```python
from build123d import *

# Parameters (mm, degrees)
F0_W         = 55
F0_H         = 46
F5_DEPTH     = 70
F1_W         = 7.25
F1_H         = 70
F6_DEPTH     = 23
F7_D         = 6
F7_DEPTH     = 15
F7_TIP       = 1.8025818571
F9_DEPTH     = 4
F10_W        = 36
F10_H        = 36
F11_DEPTH    = 4
F12_D        = 6
F12_DEPTH    = 38
F12_TIP      = 1.8025818571
F14_DEPTH    = 4
F15_T1_DEPTH = 95
F16_DEPTH    = 33
F17_DEPTH    = 10


# Not quite as in the source:
# - a fillet or chamfer that OpenCascade refuses, or shapes differently, is made with other operations: its cross-section is extruded or revolved along the edge and cut away or added


with BuildPart() as f5:
    # F0 (on Front) → F5 (new body)
    with BuildSketch(Plane.XZ):
        Rectangle(F0_W, F0_H)
    extrude(amount=-F5_DEPTH)

    # F1 (on Top) → F6 (intersect, symmetric)
    with BuildSketch(Plane.XY):
        with BuildLine():
            Line((-20.25, 0), (-13, 0))
            ThreePointArc((-13, 0), (0, 13), (13, 0))
            Line((13, 0), (20.25, 0))
            Line((20.25, 0), (20.25, 70))
            Line((20.25, 70), (-20.25, 70))
            Line((-20.25, 70), (-20.25, 0))
        make_face()
        with Locations((-23.875, 35)):
            Rectangle(F1_W, F1_H)
        with Locations((23.875, 35)):
            Rectangle(F1_W, F1_H)
    extrude(amount=F6_DEPTH, both=True, mode=Mode.INTERSECT)

    # F7
    with Locations(Plane.XZ):
        with Locations((-20.25, 0), (20.25, 0)):
            Hole(F7_D / 2, depth=F7_DEPTH)
            with Locations((0, 0, -(F7_DEPTH + F7_TIP / 2))):  # 118° drill point
                Cone(0, F7_D / 2, F7_TIP, mode=Mode.SUBTRACT)

    # F8 (on offset) → F9 (cut)
    with BuildSketch(Plane.XZ.offset(-9)):
        Polygon((-24.5, 2.4537386441), (-24.5, 2.25), (-24.5, -2.4537386441), (-20.25, -4.9074772881), (-16, -2.4537386441), (-16, 2), (-16, 2.4537386441), (-20.25, 4.9074772881), align=None)
        Polygon((-24.5, 23), (-24.5, 2.4537386441), (-20.25, 4.9074772881), (-16, 2.4537386441), (-16, 23), align=None)
        Polygon((24.5, 2.4537386441), (24.5, 23), (16, 23), (16, 2.4537386441), (16, 2), (16, -2.4537386441), (20.25, -4.9074772881), (24.5, -2.4537386441), (24.5, 2.25), align=None)
    extrude(amount=-F9_DEPTH, mode=Mode.SUBTRACT)

    # F10 (on offset) → F11 (cut)
    with BuildSketch(Plane.XZ.offset(-66)):
        Rectangle(F10_W, F10_H)
    extrude(amount=-F11_DEPTH, mode=Mode.SUBTRACT)

    # F12
    with Locations(Plane(origin=(0, 66, 0), x_dir=(1, 0, 0), z_dir=(0, 1, 0))):
        with Locations((0, 0)):
            Hole(F12_D / 2, depth=F12_DEPTH)
            with Locations((0, 0, -(F12_DEPTH + F12_TIP / 2))):  # 118° drill point
                Cone(0, F12_D / 2, F12_TIP, mode=Mode.SUBTRACT)

    # F13 (on offset) → F14 (cut)
    with BuildSketch(Plane.XZ.offset(-29)):
        Polygon((-4.25, 2.4537386441), (-4.25, 2.25), (-4.25, -2.4537386441), (0, -4.9074772881), (4.25, -2.4537386441), (4.25, 2.0686155439), (4.25, 2.4537386441), (0, 4.9074772881), align=None)
        Polygon((-4.25, 23), (-4.25, 2.4537386441), (0, 4.9074772881), (4.25, 2.4537386441), (4.25, 23), align=None)
        with BuildLine():
            ThreePointArc((23.5, 14), (22.0355339059, 17.5355339059), (18.5, 19))
            Line((18.5, 19), (13.25, 19))
            ThreePointArc((13.25, 19), (9.7144660941, 17.5355339059), (8.25, 14))
            Line((8.25, 14), (8.25, -14))
            ThreePointArc((8.25, -14), (9.7144660941, -17.5355339059), (13.25, -19))
            Line((13.25, -19), (18.5, -19))
            ThreePointArc((18.5, -19), (22.0355339059, -17.5355339059), (23.5, -14))
            Line((23.5, -14), (23.5, 14))
        make_face()
        with BuildLine():
            Line((-13.25, 19), (-18.5, 19))
            ThreePointArc((-18.5, 19), (-22.0355339059, 17.5355339059), (-23.5, 14))
            Line((-23.5, 14), (-23.5, -14))
            ThreePointArc((-23.5, -14), (-22.0355339059, -17.5355339059), (-18.5, -19))
            Line((-18.5, -19), (-13.25, -19))
            ThreePointArc((-13.25, -19), (-9.7144660941, -17.5355339059), (-8.25, -14))
            Line((-8.25, -14), (-8.25, 14))
            ThreePointArc((-8.25, 14), (-9.7144660941, 17.5355339059), (-13.25, 19))
        make_face()
    extrude(amount=-F14_DEPTH, mode=Mode.SUBTRACT)

    # F15: fillet of radius 5 on 4 edges, made by hand

    # F15_s2 → F15_t1 (cut)
    with BuildSketch(Plane.XZ.offset(-82.5)):
        with BuildLine():
            ThreePointArc((-22.5, 23), (-26.0355339059, 21.5355339059), (-27.5, 18))
            Line((-27.5, 18), (-27.5, 23))
            Line((-27.5, 23), (-22.5, 23))
        make_face()
        with BuildLine():
            ThreePointArc((22.5, 23), (26.0355339059, 21.5355339059), (27.5, 18))
            Line((27.5, 18), (27.5, 23))
            Line((27.5, 23), (22.5, 23))
        make_face()
        with BuildLine():
            ThreePointArc((-22.5, -23), (-26.0355339059, -21.5355339059), (-27.5, -18))
            Line((-27.5, -18), (-27.5, -23))
            Line((-27.5, -23), (-22.5, -23))
        make_face()
        with BuildLine():
            ThreePointArc((22.5, -23), (26.0355339059, -21.5355339059), (27.5, -18))
            Line((27.5, -18), (27.5, -23))
            Line((27.5, -23), (22.5, -23))
        make_face()
    extrude(amount=F15_T1_DEPTH, mode=Mode.SUBTRACT)

    # F13 (on offset) → F16 (cut)
    with BuildSketch(Plane.XZ.offset(-29)):
        with BuildLine():
            ThreePointArc((23.5, 14), (22.0355339059, 17.5355339059), (18.5, 19))
            Line((18.5, 19), (13.25, 19))
            ThreePointArc((13.25, 19), (9.7144660941, 17.5355339059), (8.25, 14))
            Line((8.25, 14), (8.25, -14))
            ThreePointArc((8.25, -14), (9.7144660941, -17.5355339059), (13.25, -19))
            Line((13.25, -19), (18.5, -19))
            ThreePointArc((18.5, -19), (22.0355339059, -17.5355339059), (23.5, -14))
            Line((23.5, -14), (23.5, 14))
        make_face()
        with BuildLine():
            Line((-13.25, 19), (-18.5, 19))
            ThreePointArc((-18.5, 19), (-22.0355339059, 17.5355339059), (-23.5, 14))
            Line((-23.5, 14), (-23.5, -14))
            ThreePointArc((-23.5, -14), (-22.0355339059, -17.5355339059), (-18.5, -19))
            Line((-18.5, -19), (-13.25, -19))
            ThreePointArc((-13.25, -19), (-9.7144660941, -17.5355339059), (-8.25, -14))
            Line((-8.25, -14), (-8.25, 14))
            ThreePointArc((-8.25, 14), (-9.7144660941, 17.5355339059), (-13.25, 19))
        make_face()
    extrude(amount=-F16_DEPTH, mode=Mode.SUBTRACT)

    # F13 (on offset) → F17 (cut)
    with BuildSketch(Plane.XZ.offset(-29)):
        with BuildLine():
            ThreePointArc((23.5, 14), (22.0355339059, 17.5355339059), (18.5, 19))
            Line((18.5, 19), (13.25, 19))
            ThreePointArc((13.25, 19), (9.7144660941, 17.5355339059), (8.25, 14))
            Line((8.25, 14), (8.25, -14))
            ThreePointArc((8.25, -14), (9.7144660941, -17.5355339059), (13.25, -19))
            Line((13.25, -19), (18.5, -19))
            ThreePointArc((18.5, -19), (22.0355339059, -17.5355339059), (23.5, -14))
            Line((23.5, -14), (23.5, 14))
        make_face()
        with BuildLine():
            Line((-13.25, 19), (-18.5, 19))
            ThreePointArc((-18.5, 19), (-22.0355339059, 17.5355339059), (-23.5, 14))
            Line((-23.5, 14), (-23.5, -14))
            ThreePointArc((-23.5, -14), (-22.0355339059, -17.5355339059), (-18.5, -19))
            Line((-18.5, -19), (-13.25, -19))
            ThreePointArc((-13.25, -19), (-9.7144660941, -17.5355339059), (-8.25, -14))
            Line((-8.25, -14), (-8.25, 14))
            ThreePointArc((-8.25, 14), (-9.7144660941, 17.5355339059), (-13.25, 19))
        make_face()
    extrude(amount=F17_DEPTH, mode=Mode.SUBTRACT)


solid = f5.part
```
Geometry check sheet. Reference: the model listing, model coordinates, mm. A direction names the side the tool comes from. Give positions to 0.01 mm unless a question says otherwise; leave off trailing zeros. Order: outer loops, then holes, each group sorted by start corner. A loop starts at its lowest first (then second) coordinate and runs counter-clockwise, first axis right, second up. Notation, with made-up numbers: (-10, 45) - (-5, 45) arc R5 cw to (-5, 54) - close; hole circle Ø5 at (-32, 10.5). An arc over 180 degrees is marked (long way). Write item = value, one per line. Start each with the question number.
1) Section check C-C (x = -6.5). Enter the section's corners in (y, z), then the cut area to 3 significant figures.
2) Section check A-A (z = -11.5). Enter the section's corners in (x, y).
3) Gauge pin test, flat ends, axial feed: pin 1 Ø4 at (x, z) = (1.5, 7) entering from -Y; pin 2 Ø8 at (x, z) = (-10.5, -7) entering from +Y; pin 3 Ø4.5 at (x, z) = (17.5, -4.5) entering from +Y; pin 4 Ø5 at (x, z) = (0, 0) entering from -Y. Record the tip position at first contact, or that the pin passes through.
4) Access from +Z, -Z, +X, -X, +Y, -Y to the whole of each face (thin tool, end or side, straight path). Record for faces 1 (the flat face through (-18, 68, 0)), 2 (the flat face through (-16, 62, 0)), 3 (the flat face through (20, 9, 9)).
5) Section check D-D (z = 20.5). Enter the section's corners in (x, y).
6) Scan lines: L1, parallel to X at y = 34, z = -8; L2, parallel to X at y = 14.2, z = 0; L3, parallel to X at y = 32.5, z = 4. Record each from-to range of solid material in increasing order.
7) Draft check along X on faces 4 (the flat face through (17, 0, 0)), 5 (the flat face through (2.095, 30.972, -3.698)), 6 (the flat face through (-16, 11, 10)), 7 (the flat face through (27.5, 35, 0)). Enter one of: released by +X, released by -X, zero draft, split by the parting line, or undercut.
8) Section check B-B (z = 12). Count the separate pieces of the cut face and the enclosed holes in it, then the cut area to 3 significant figures.
Geometry check:
q1.outline = (11.26, -23) - (70, -23) - (70, -18) - (66, -18) - (66, 18) - (70, 18) - (70, 23) - (11.26, 23) - close
q1.area = 2,560 mm2
q2.outline = (-27.5, 0) - (-13, 0) arc R13 cw to (13, 0) - (27.5, 0) - (27.5, 70) - (18, 70) - (18, 66) - (-18, 66) - (-18, 70) - (-27.5, 70) - close; hole (-23.5, 19) - (-8.25, 19) - (-8.25, 62) - (-23.5, 62) - close; hole (8.25, 19) - (23.5, 19) - (23.5, 62) - (8.25, 62) - close
q3.pin_1 = 12.52
q3.pin_2 = 66
q3.pin_3 = 70
q3.pin_4 = 12.76
q4.face_1 = +Y
q4.face_2 = none
q4.face_3 = +Z
q5.outline = (-26.83, 0) - (-13, 0) arc R13 cw to (13, 0) - (26.83, 0) - (26.83, 70) - (-26.83, 70) - close; hole (-24.5, 9) - (-16, 9) - (-16, 13) - (-24.5, 13) - close; hole (-4.25, 29) - (4.25, 29) - (4.25, 33) - (-4.25, 33) - close; hole (16, 9) - (24.5, 9) - (24.5, 13) - (16, 13) - close
q6.L1 = -27.5 to -23.5, -8.25 to 8.25, 23.5 to 27.5
q6.L2 = -27.5 to -23.25, -17.25 to 17.25, 23.25 to 27.5
q6.L3 = -27.5 to -23.5, -8.25 to -4.25, 4.25 to 8.25, 23.5 to 27.5
q7.face_4 = zero draft
q7.face_5 = undercut
q7.face_6 = undercut
q7.face_7 = released by +X
q8.separate_pieces = 1
q8.enclosed_holes = 5
q8.area = 2,030 mm2
